CAD build for the part. Positions are in the model's coordinates, mm. A direction names the side the tool comes from. Give positions to 0.01 mm unless a question says otherwise; leave off trailing zeros. Order: outer loops, then holes, each group sorted by start corner. A loop starts at its lowest first (then second) coordinate and runs counter-clockwise, first axis right, second up.
Item 1: Two-plate mould, pull along Z, no slides. Class faces 1 (the cylindrical face through (-24.275, 0.739, -13.697)), 2 (the flat face through (0, 1, 20.5)), 3 (the flat face through (30, 1, 22)): released by +Z, released by -Z, zero draft, split by the parting line, or undercut.
Item 2: Band-saw the part on C-C on x = 24. Give the cut face in (y, z), plus the area to 3 significant figures.
Item 3: Band-saw the part on D-D on y = 1.2. Count the separate pieces of the cut face and the enclosed holes in it, plus the area to 3 significant figures.
Item 4: Which spindle directions (+Z, -Z, +X, -X, +Y, -Y) get a long thin tool onto all of the face, cutting with end or side? Do faces 4 (the cylindrical face through (16.197, 0.739, -21.775)), 5 (the cylindrical face through (-16.197, 0.739, 21.775)), 6 (the cylindrical face through (24.275, 0.739, 13.697)), 7 (the cylindrical face through (-24.35, 0.74, 13.79)). Say none if no direction does.
Item 5: Band-saw the part on A-A on z = -22.5. Give the cut face in (x, y).
Item 6: Band-saw the part on B-B on x = 15.25. Give the cut face in (y, z).
Item 7: Wall check: L1, parallel to X at y = 0.6, z = 15.25; L2, parallel to X at y = 0.25, z = 24; L3, parallel to X at y = 0.7, z = -22.5. Give the ranges that are in metal, low to high.
```python
from build123d import *

# Parameters (mm, degrees)
SKETCH1_W           = 60
SKETCH1_H           = 55
BOSS_EXTRUDE1_DEPTH = 1.5
SKETCH2_R           = 3.1
CUT_EXTRUDE1_DEPTH  = 41.724685389
FILLET1_R           = 3
SKETCH4_W           = 37
SKETCH4_H           = 7
SKETCH4_W_2         = 7
SKETCH4_H_2         = 32
CUT_EXTRUDE2_DEPTH  = 41.724685389
FILLET2_R           = 6
FILLET3_R           = 3
SKETCH5_R           = 1.1
CUT_EXTRUDE3_DEPTH  = 41.724685533


with BuildPart() as part:
    # Sketch1 → Boss-Extrude1 (new body)
    with BuildSketch(Plane(origin=(0, 0, 0), x_dir=(1, 0, 0), z_dir=(0, 1, 0))):
        Rectangle(SKETCH1_W, SKETCH1_H)
    extrude(amount=BOSS_EXTRUDE1_DEPTH)

    # Sketch2 → Cut-Extrude1 (cut, through all)
    with BuildSketch(Plane(origin=(0, 1.5, 0), x_dir=(1, 0, 0), z_dir=(0, 1, 0))):
        with Locations(Location((-25, 22.5, 0), (0, 0, 270))):
            Circle(SKETCH2_R)
        with Locations(Location((25, 22.5, 0), (0, 0, 270))):
            Circle(SKETCH2_R)
        with Locations(Location((-25, -22.5, 0), (0, 0, 270))):
            Circle(SKETCH2_R)
        with Locations(Location((25, -22.5, 0), (0, 0, 270))):
            Circle(SKETCH2_R)
    extrude(amount=-CUT_EXTRUDE1_DEPTH, mode=Mode.SUBTRACT)

    # Fillet1
    fillet1_edges = [part.edges().sort_by_distance(p)[0] for p in [
        (-30, 0.75, -27.5),
        (30, 0.75, -27.5),
        (30, 0.75, 27.5),
        (-30, 0.75, 27.5),
    ]]
    fillet(fillet1_edges, radius=FILLET1_R)

    # Sketch4 → Cut-Extrude2 (cut, through all)
    with BuildSketch(Plane(origin=(0, 1.5, 0), x_dir=(1, 0, 0), z_dir=(0, 1, 0))):
        with Locations((0, 24)):
            Rectangle(SKETCH4_W, SKETCH4_H)
        with Locations((-26.5, 0)):
            Rectangle(SKETCH4_W_2, SKETCH4_H_2)
        with Locations((0, -24)):
            Rectangle(SKETCH4_W, SKETCH4_H)
        with Locations((26.5, 0)):
            Rectangle(SKETCH4_W_2, SKETCH4_H_2)
    extrude(amount=-CUT_EXTRUDE2_DEPTH, mode=Mode.SUBTRACT)

    # Fillet2
    fillet2_edges = [part.edges().sort_by_distance(p)[0] for p in [
        (-18.5, 0.75, -20.5),
        (18.5, 0.75, -20.5),
        (-23, 0.75, -16),
        (-23, 0.75, 16),
        (-18.5, 0.75, 20.5),
        (18.5, 0.75, 20.5),
        (23, 0.75, -16),
        (23, 0.75, 16),
    ]]
    fillet(fillet2_edges, radius=FILLET2_R)

    # Fillet3
    fillet3_edges = [part.edges().sort_by_distance(p)[0] for p in [
        (30, 0.75, -16),
        (18.5, 0.75, -27.5),
        (30, 0.75, 16),
        (18.5, 0.75, 27.5),
        (-18.5, 0.75, 27.5),
        (-30, 0.75, 16),
        (-18.5, 0.75, -27.5),
        (-30, 0.75, -16),
    ]]
    fillet(fillet3_edges, radius=FILLET3_R)

    # Sketch5 → Cut-Extrude3 (cut, through all)
    with BuildSketch(Plane(origin=(0, 1.5, 0), x_dir=(1, 0, 0), z_dir=(0, 1, 0))):
        with Locations(Location((-15.25, 15.25, 0), (0, 0, 270))):
            Circle(SKETCH5_R)
        with Locations(Location((15.25, 15.25, 0), (0, 0, 270))):
            Circle(SKETCH5_R)
        with Locations(Location((-15.25, -15.25, 0), (0, 0, 270))):
            Circle(SKETCH5_R)
        with Locations(Location((15.25, -15.25, 0), (0, 0, 270))):
            Circle(SKETCH5_R)
    extrude(amount=-CUT_EXTRUDE3_DEPTH, mode=Mode.SUBTRACT)


solid = part.part
```
The answers:
1. face 1: undercut
1. face 2: released by +Z
1. face 3: zero draft
2. outline: (0, -27.5) - (1.5, -27.5) - (1.5, -25.43) - (0, -25.43) - close; (0, -19.57) - (1.5, -19.57) - (1.5, -13.32) - (0, -13.32) - close; (0, 13.32) - (1.5, 13.32) - (1.5, 19.57) - (0, 19.57) - close; (0, 25.43) - (1.5, 25.43) - (1.5, 27.5) - (0, 27.5) - close
2. area: 24.9 mm2
3. separate pieces: 1
3. enclosed holes: 8
3. area: 2,240 mm2
4. face 4: -Z, +Y, -Y
4. face 5: +Z, +Y, -Y
4. face 6: +X, +Y, -Y
4. face 7: -X, +Y, -Y
5. outline: (-30, 0) - (-28.1, 0) - (-28.1, 1.5) - (-30, 1.5) - close; (-21.9, 0) - (-16.97, 0) - (-16.97, 1.5) - (-21.9, 1.5) - close; (16.97, 0) - (21.9, 0) - (21.9, 1.5) - (16.97, 1.5) - close; (28.1, 0) - (30, 0) - (30, 1.5) - (28.1, 1.5) - close
6. outline: (0, -21.17) - (1.5, -21.17) - (1.5, -16.35) - (0, -16.35) - close; (0, -14.15) - (1.5, -14.15) - (1.5, 14.15) - (0, 14.15) - close; (0, 16.35) - (1.5, 16.35) - (1.5, 21.17) - (0, 21.17) - close
7. L1: x = -26.1 to -16.35, -14.15 to 14.15, 16.35 to 26.1
7. L2: x = -30 to -27.71, -22.29 to -17.95, 17.95 to 22.29, 27.71 to 30
7. L3: x = -30 to -28.1, -21.9 to -16.97, 16.97 to 21.9, 28.1 to 30
